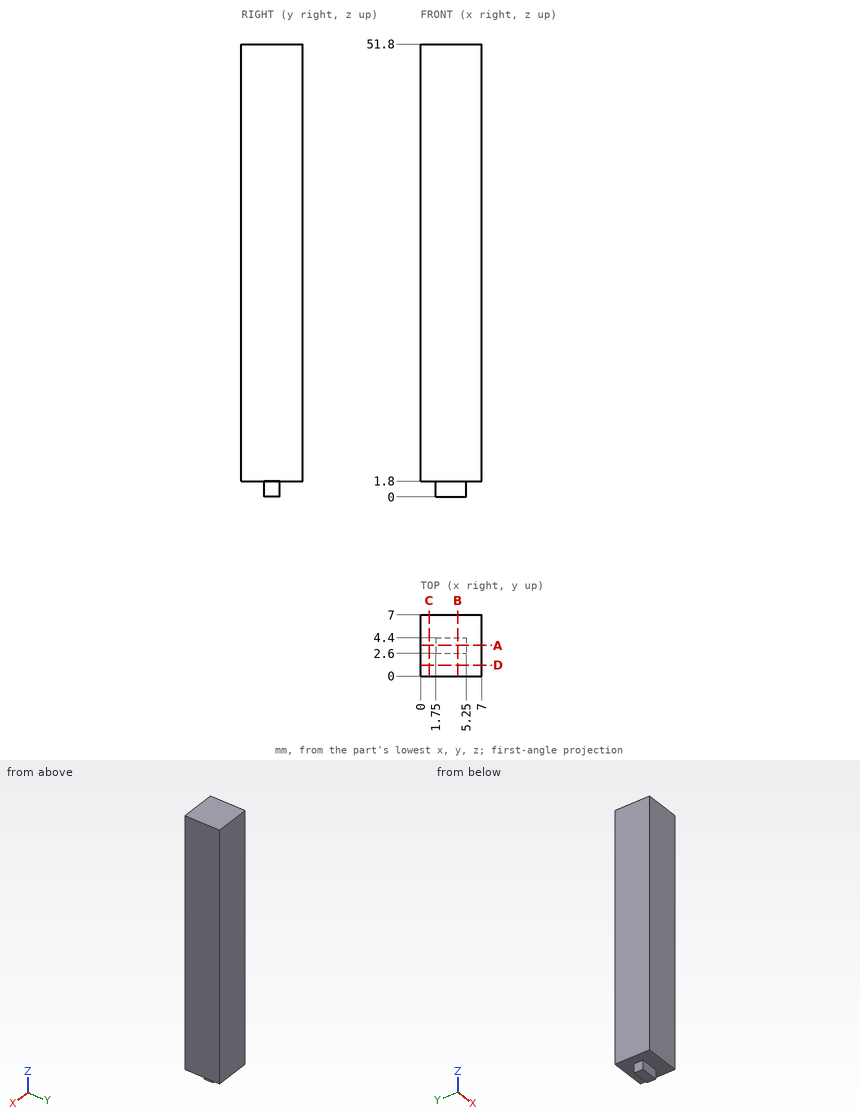
Job drawing, mm, ordinate dimensions from the low corner. One solid piece. Coordinates: 2 decimals unless noted, no trailing zeros. Order: outer loops, then holes, each group sorted by start corner. A loop starts at its lowest first (then second) coordinate and runs counter-clockwise, first axis right, second up. Notation, with made-up numbers: (-5, 0) - (22, 0) arc R27 ccw to (22, 19) - close; hole circle Ø5 at (32, 44). An arc over 180 degrees is marked (long way). Return JSON: item names as keys, results as strings. Group by question number.
1) Saw through at B-B, the plane x = 4.25. Write the cut outline in (y, z), plus the area to 3 significant figures.
2) Probe line 1 (Z direction, x = 5.75, y = 3). List the from-to ranges inside material, lowest first. Write a range as from..to.
3) Saw through at A-A, the plane y = 3.5. Write the cut outline in (x, z), plus the area to 3 significant figures.
4) Saw through at C-C, the plane x = 1. Write the cut outline in (y, z), plus the area to 3 significant figures.
5) Flat gauge pins, fed straight in: P1, Ø1.5, axis at x = 1, z = 34, coming from the -Y side; P2, Ø1.4, axis at x = 3, z = 0.5, coming from the -Y side; P3, Ø0.5, axis at x = 3.5, z = 1.5, coming from the +Y side; P4, Ø1.4, axis at y = 3.5, z = 1, coming from the -X side. Where does each tip first touch, or does it go through?
Values found:
{
 "1": {"outline": "(0, 1.8) - (2.6, 1.8) - (2.6, 0) - (4.4, 0) - (4.4, 1.8) - (7, 1.8) - (7, 51.8) - (0, 51.8) - close", "area": "353 mm²"},
 "2": {"line 1": "z = 1.8..51.8"},
 "3": {"outline": "(0, 1.8) - (1.75, 1.8) - (1.75, 0) - (5.25, 0) - (5.25, 1.8) - (7, 1.8) - (7, 51.8) - (0, 51.8) - close", "area": "356 mm²"},
 "4": {"outline": "(0, 1.8) - (7, 1.8) - (7, 51.8) - (0, 51.8) - close", "area": "350 mm²"},
 "5": {"P1": "stops at y = 0", "P2": "stops at y = 2.6", "P3": "stops at y = 4.4", "P4": "stops at x = 1.75"}
}
